Source: CAD feature listing. Evaluate the final solid. Frame: model axes, mm. Face numbers are marked on the shaded views. Give positions to 0.01 mm unless a question says otherwise; leave off trailing zeros. Write each loop counter-clockwise with the first axis right and the second up, starting at its lowest first coordinate (ties: lowest second). Pieces come first, ordered by that corner, then holes. Notation, with made-up numbers: M 54.5,-9 L 68.5,-9 A26 ccw 68.5,21 Z; hole C 38,13 d1. An arc over 180 degrees is marked long. Return JSON: item names as keys, results as strings.
```python
from build123d import *

# Parameters (mm, degrees)
F0_R     = 16.5
F1_DEPTH = 17
F2_R     = 15
F3_DEPTH = 15
F4_R     = 1.4
F5_DEPTH = 20
F7_DEPTH = 2


with BuildPart() as f1:
    # F0 (on Top) → F1 (new body)
    with BuildSketch(Plane.XY):
        Circle(F0_R)
    extrude(amount=F1_DEPTH)

    # F2 (on Top) → F3 (cut)
    with BuildSketch(Plane.XY):
        Circle(F2_R)
    extrude(amount=F3_DEPTH, mode=Mode.SUBTRACT)

    # F4 (on Right) → F5 (cut, symmetric)
    with BuildSketch(Plane.YZ):
        with Locations((0, 9.5)):
            Circle(F4_R)
    extrude(amount=F5_DEPTH, both=True, mode=Mode.SUBTRACT)

    # F6 (on face) → F7 (cut)
    with BuildSketch(Plane.XY.offset(17)):
        Polygon((1.5, 6), (-1.5, 6), (-1.5, 1.5), (0.375, 1.5), align=None)
        Polygon((1.5, 1.5), (1.5, 6), (0.375, 1.5), align=None)
        Polygon((0.375, 1.5), (-1.5, 1.5), (-1.5, -0.375), (0, 0), align=None)
        Polygon((-1.5, -0.375), (-1.5, 1.5), (-6, 1.5), (-6, -1.5), align=None)
        Polygon((6, 1.5), (1.5, 1.5), (1.5, 0.375), align=None)
        Polygon((1.5, 0.375), (1.5, 1.5), (0.375, 1.5), (0, 0), align=None)
        Polygon((0, 0), (-1.5, -0.375), (-1.5, -1.5), (-0.375, -1.5), align=None)
        Polygon((-1.5, -1.5), (-1.5, -0.375), (-6, -1.5), align=None)
        Polygon((6, 1.5), (1.5, 0.375), (1.5, -1.5), (6, -1.5), align=None)
        Polygon((1.5, -1.5), (1.5, 0.375), (0, 0), (-0.375, -1.5), align=None)
        Polygon((-0.375, -1.5), (-1.5, -1.5), (-1.5, -6), align=None)
        Polygon((1.5, -6), (1.5, -1.5), (-0.375, -1.5), (-1.5, -6), align=None)
    extrude(amount=-F7_DEPTH, mode=Mode.SUBTRACT)


solid = f1.part
```
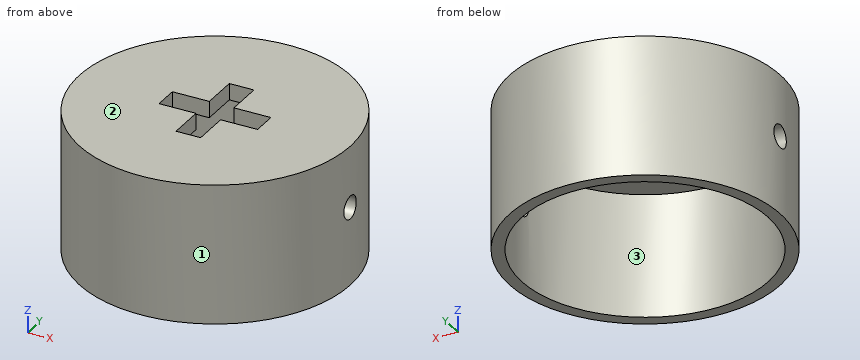
1) Draft query along Y for the marked faces 1, 2 and 3. Return one class per face: released by +Y, released by -Y, zero draft, split by the parting line, or undercut.
Numbers:
{"face 1": "split by the parting line", "face 2": "zero draft", "face 3": "undercut"}
2) Cut plane A-A, the plane x = 0. Return the cut outline in (y, z).
Numbers:
{"outline": "M -16.5,0 L -15,0 L -15,15 L -6,15 L -6,17 L -16.5,17 Z; M 6,15 L 15,15 L 15,0 L 16.5,0 L 16.5,17 L 6,17 Z"}
3) Cut plane C-C, the plane y = 4.5. Return the cut outline in (x, z).
Numbers:
{"outline": "M -15.87,0 L -14.31,0 L -14.31,15 L -1.5,15 L -1.5,17 L -15.87,17 Z; M 1.5,15 L 14.31,15 L 14.31,0 L 15.87,0 L 15.87,17 L 1.5,17 Z"}
4) Cut plane B-B, the plane y = 0. Return the cut outline in (x, z).
Numbers:
{"outline": "M -16.5,0 L -15,0 L -15,8.1 L -16.5,8.1 Z; M -16.5,10.9 L -15,10.9 L -15,15 L -6,15 L -6,17 L -16.5,17 Z; M 6,15 L 15,15 L 15,10.9 L 16.5,10.9 L 16.5,17 L 6,17 Z; M 15,0 L 16.5,0 L 16.5,8.1 L 15,8.1 Z"}
5) Contact query for flat-ended pins moving along their axis: pin 1 Ø10 at (x, z) = (9, 3) entering from +Y; pin 2 Ø2 at (y, z) = (8, 12.5) entering from -X; pin 3 Ø1.6 at (y, z) = (3.5, 16) entering from -X. Output: stop coordinate, or through.
Numbers:
{"pin 1": "stops at y = 16.01", "pin 2": "stops at x = -14.94", "pin 3": "stops at x = -16.28"}
6) Cut plane D-D, the plane z = 1.5. Return the cut outline in (x, y), then the cut area to 3 significant figures.
Numbers:
{"outline": "C 0,0 d33; hole C 0,0 d30", "area": "148 mm²"}
7) Line query: line 1 (X direction, y = 0, z = 11.75); line 2 (Y direction, x = -8.5, z = 3.5). Output: solid intervals per line, ascending. Write a range as [from, to].
Numbers:
{"line 1": "x = [-16.5, -15], [15, 16.5]", "line 2": "y = [-14.14, -12.36], [12.36, 14.14]"}
